The figure shows three views and two pictorial views of one solid part (mm, origin at its lowest corner). Answer the questions. Give positions to 0.01 mm unless a question says otherwise; leave off trailing zeros. Order: outer loops, then holes, each group sorted by start corner. A loop starts at its lowest first (then second) coordinate and runs counter-clockwise, first axis right, second up. Notation, with made-up numbers: M 8,-2.75 L 19,-2.75 A19 cw 19,28.25 Z; hole C 55.25,-16.5 d7. An arc over 180 degrees is marked long. One line per item, written item: value. Start each with the question number.
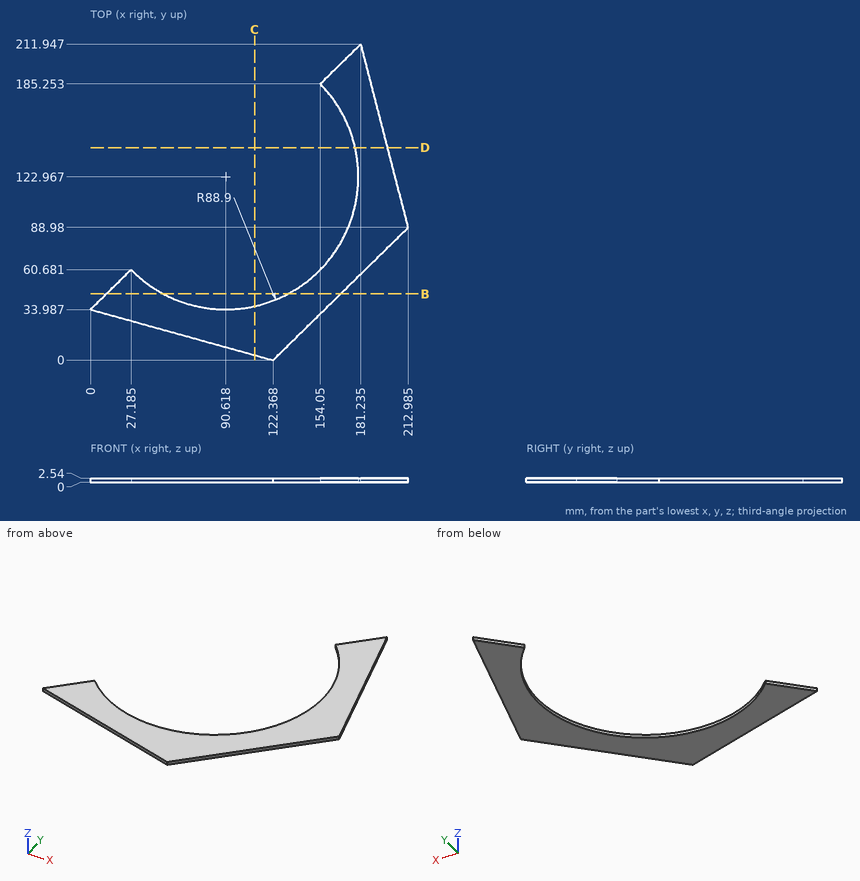
Q1. Find section B-B, the plane y = 44.5. Give the vertices of the cut face in (x, z) (1 decimal).
Q2. Find section D-D, the plane y = 142.5. Give the vertices of the cut face in (x, z) (1 decimal).
Q3. Find section C-C, the plane x = 110. Give the vertices of the cut face in (y, z) (1 decimal).
Q4. This flat-tipped pin is pushed along its axis until it touches: pin 1 (1.5 mm diameter, centred on y = 137, z = 2, fed in from +X). Where does it stop, or does it pass through?
Q5. Consider probe 1 along X at (y, z) = (168, 2.2); probe 2 along X at (y, z) = (80, 1.65) (1 decimal); probe 3 along Y at (x, z) = (104, 1.15). Determine where each line is inside the solid, lowest interval first.
Evaluation:
1. outline: M 10.7,0 L 48.8,0 L 48.8,2.5 L 10.7,2.5 Z; M 132.4,0 L 167.7,0 L 167.7,2.5 L 132.4,2.5 Z
2. outline: M 177.3,0 L 199.2,0 L 199.2,2.5 L 177.3,2.5 Z
3. outline: M 3.4,0 L 36.2,0 L 36.2,2.5 L 3.4,2.5 Z
4. pin 1: x = 200.78
5. probe 1: 167.27 to 192.58
5. probe 2: 168.4 to 203.8
5. probe 3: 5.1 to 35.08
